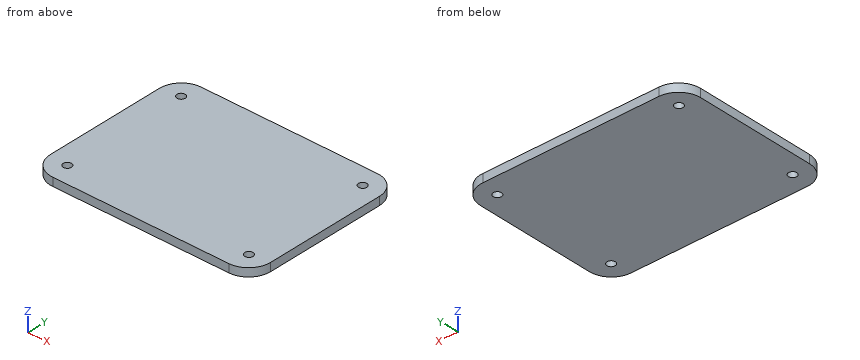
from build123d import *

# Parameters (mm, degrees)
SKETCH1_W           = 80
SKETCH1_H           = 60
BOSS_EXTRUDE1_DEPTH = 3
FILLET1_R           = 8
SKETCH2_R           = 1.5
CUT_EXTRUDE1_DEPTH  = 3


with BuildPart() as part:
    # Sketch1 → Boss-Extrude1 (new body)
    with BuildSketch(Plane.XY):
        Rectangle(SKETCH1_W, SKETCH1_H)
    extrude(amount=BOSS_EXTRUDE1_DEPTH)

    # Fillet1
    fillet1_edges = [part.edges().sort_by_distance(p)[0] for p in [
        (-40, 30, 1.5),
        (40, 30, 1.5),
        (40, -30, 1.5),
        (-40, -30, 1.5),
    ]]
    fillet(fillet1_edges, radius=FILLET1_R)

    # Sketch2 → Cut-Extrude1 (cut)
    with BuildSketch(Plane(origin=(0, 0, 0), x_dir=(-1, 0, 0), z_dir=(0, 0, -1))):
        with Locations((33, -23)):
            Circle(SKETCH2_R)
        with Locations((33, 23)):
            Circle(SKETCH2_R)
        with Locations((-33, 23)):
            Circle(SKETCH2_R)
        with Locations((-33, -23)):
            Circle(SKETCH2_R)
    extrude(amount=-CUT_EXTRUDE1_DEPTH, mode=Mode.SUBTRACT)


solid = part.part
Work out the finished part from the listing and answer in its coordinate system (mm). Give positions to 0.01 mm unless a question says otherwise; leave off trailing zeros. Write each loop counter-clockwise with the first axis right and the second up, starting at its lowest first coordinate (ties: lowest second). Pieces come first, ordered by that corner, then holes. Notation, with made-up numbers: (68, 6.25) - (78, 6.25) arc R23 ccw to (78, 27.25) - close; hole circle Ø10 at (41, 23). An arc over 180 degrees is marked (long way). One line per item, written item: value. Start each with the question number.
1. Find section A-A (z = 0.65). Write down the section's boundary in (x, y), then the cut area to 3 significant figures.
2. Consider probe 1 along Y at (x, z) = (-33, 1.65); probe 2 along X at (y, z) = (-22.5, 2.6). Determine where each line is inside the solid, lowest interval first.
3. Find section C-C (y = -23). Write down the section's boundary in (x, z).
4. Find section B-B (x = 33). Write down the section's boundary in (y, z).
Geometry results:
1. outline: (-40, -22) arc R8 ccw to (-32, -30) - (32, -30) arc R8 ccw to (40, -22) - (40, 22) arc R8 ccw to (32, 30) - (-32, 30) arc R8 ccw to (-40, 22) - close; hole circle Ø3 at (-33, -23); hole circle Ø3 at (-33, 23); hole circle Ø3 at (33, -23); hole circle Ø3 at (33, 23)
1. area: 4,720 mm2
2. probe 1: -29.94 to -24.5, -21.5 to 21.5, 24.5 to 29.94
2. probe 2: -39.98 to -34.41, -31.59 to 31.59, 34.41 to 39.98
3. outline: (-39.94, 0) - (-34.5, 0) - (-34.5, 3) - (-39.94, 3) - close; (-31.5, 0) - (31.5, 0) - (31.5, 3) - (-31.5, 3) - close; (34.5, 0) - (39.94, 0) - (39.94, 3) - (34.5, 3) - close
4. outline: (-29.94, 0) - (-24.5, 0) - (-24.5, 3) - (-29.94, 3) - close; (-21.5, 0) - (21.5, 0) - (21.5, 3) - (-21.5, 3) - close; (24.5, 0) - (29.94, 0) - (29.94, 3) - (24.5, 3) - close
